CAD build for the part. Positions are in the model's coordinates, mm. Face numbers are marked on the shaded views. Coordinates: 2 decimals unless noted, no trailing zeros. Order: outer loops, then holes, each group sorted by start corner. A loop starts at its lowest first (then second) coordinate and runs counter-clockwise, first axis right, second up. Notation, with made-up numbers: (58.5, 3.5) - (66.5, 3.5) arc R13 ccw to (66.5, 7.5) - close; hole circle Ø1 at (82.25, -4.75). An arc over 180 degrees is marked (long way). Return JSON: item names as keys, results as strings.
from build123d import *

# Parameters (mm, degrees)
SKETCH2_R           = 20
SKETCH2_R_2         = 10
BOSS_EXTRUDE1_DEPTH = 110
SKETCH3_R           = 30
BOSS_EXTRUDE2_DEPTH = 10
CUT_EXTRUDE1_START  = -10
SKETCH4_R           = 10
CUT_EXTRUDE1_DEPTH  = 10


with BuildPart() as part:
    # Sketch2 → Boss-Extrude1 (new body)
    with BuildSketch(Plane(origin=(0, 0, 0), x_dir=(0, 1, 0), z_dir=(0, 0, 1))):
        with Locations(Location((0, 0, 0), (0, 0, 270))):
            Circle(SKETCH2_R)
        with Locations(Location((0, 0, 0), (0, 0, 270))):
            Circle(SKETCH2_R_2, mode=Mode.SUBTRACT)
    extrude(amount=BOSS_EXTRUDE1_DEPTH)

    # Sketch3 → Boss-Extrude2 (add)
    with BuildSketch(Plane(origin=(0, 0, 0), x_dir=(0, 1, 0), z_dir=(0, 0, 1))):
        with Locations(Location((0, 0, 0), (0, 0, 270))):
            Circle(SKETCH3_R)
    extrude(amount=BOSS_EXTRUDE2_DEPTH)

    # Sketch4 → Cut-Extrude1 (cut)
    with BuildSketch(Plane.XY.offset(10).offset(CUT_EXTRUDE1_START)):
        Circle(SKETCH4_R)
    extrude(amount=CUT_EXTRUDE1_DEPTH, mode=Mode.SUBTRACT)


solid = part.part
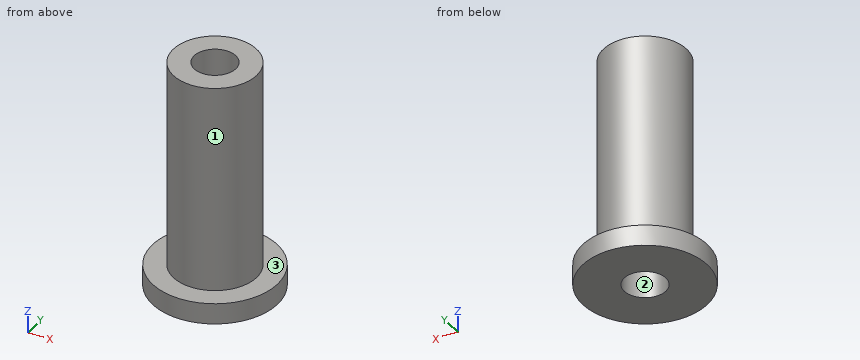
Item 1: Drop flat-ended pins along their axis: P1, Ø1, axis at y = -17.5, z = 35.5, coming from the +X side; P2, Ø5, axis at x = -21.5, y = -3.5, coming from the -Z side; P3, Ø1.5, axis at y = -14.5, z = 94, coming from the +X side; P4, Ø6, axis at y = 7, z = 62.5, coming from the +X side. Give the stop position or say it passes through.
Findings below:
{"P1": "stops at x = 10.54", "P2": "stops at z = 0", "P3": "stops at x = 14.52", "P4": "stops at x = 19.6"}
Item 2: Wall check: L1, parallel to Y at x = 0, z = 73.5; L2, parallel to X at y = -0.5, z = 102; L3, parallel to Z at x = -22, y = 18. Give the ranges that are in metal, low to high. Write a range as [from, to].
Findings below:
{"L1": "y = [-20, -10], [10, 20]", "L2": "x = [-19.99, -9.99], [9.99, 19.99]", "L3": "z = [0, 10]"}
Item 3: Band-saw the part on C-C, the plane z = 62.5. List the corners of the cut face in (x, y).
Findings below:
{"outline": "circle Ø40 at (0, 0); hole circle Ø20 at (0, 0)"}
Item 4: Band-saw the part on A-A, the plane y = 0. List the corners of the cut face in (x, z).
Findings below:
{"outline": "(-30, 0) - (-10, 0) - (-10, 110) - (-20, 110) - (-20, 10) - (-30, 10) - close; (10, 0) - (30, 0) - (30, 10) - (20, 10) - (20, 110) - (10, 110) - close"}
Item 5: Mould opens along X. For the marked faces 1, 2 and 3 say: released by +X, released by -X, zero draft, split by the parting line, or undercut.
Findings below:
{"face 1": "split by the parting line", "face 2": "undercut", "face 3": "zero draft"}
Item 6: Band-saw the part on D-D, the plane x = 17.5. List the corners of the cut face in (y, z), then the cut area to 3 significant figures.
Findings below:
{"outline": "(-24.37, 0) - (24.37, 0) - (24.37, 10) - (9.68, 10) - (9.68, 110) - (-9.68, 110) - (-9.68, 10) - (-24.37, 10) - close", "area": "2,420 mm²"}
Item 7: Band-saw the part on B-B, the plane x = 0.5. List the corners of the cut face in (y, z), then the cut area to 3 significant figures.
Findings below:
{"outline": "(-30, 0) - (-9.99, 0) - (-9.99, 110) - (-19.99, 110) - (-19.99, 10) - (-30, 10) - close; (9.99, 0) - (30, 0) - (30, 10) - (19.99, 10) - (19.99, 110) - (9.99, 110) - close", "area": "2,400 mm²"}
